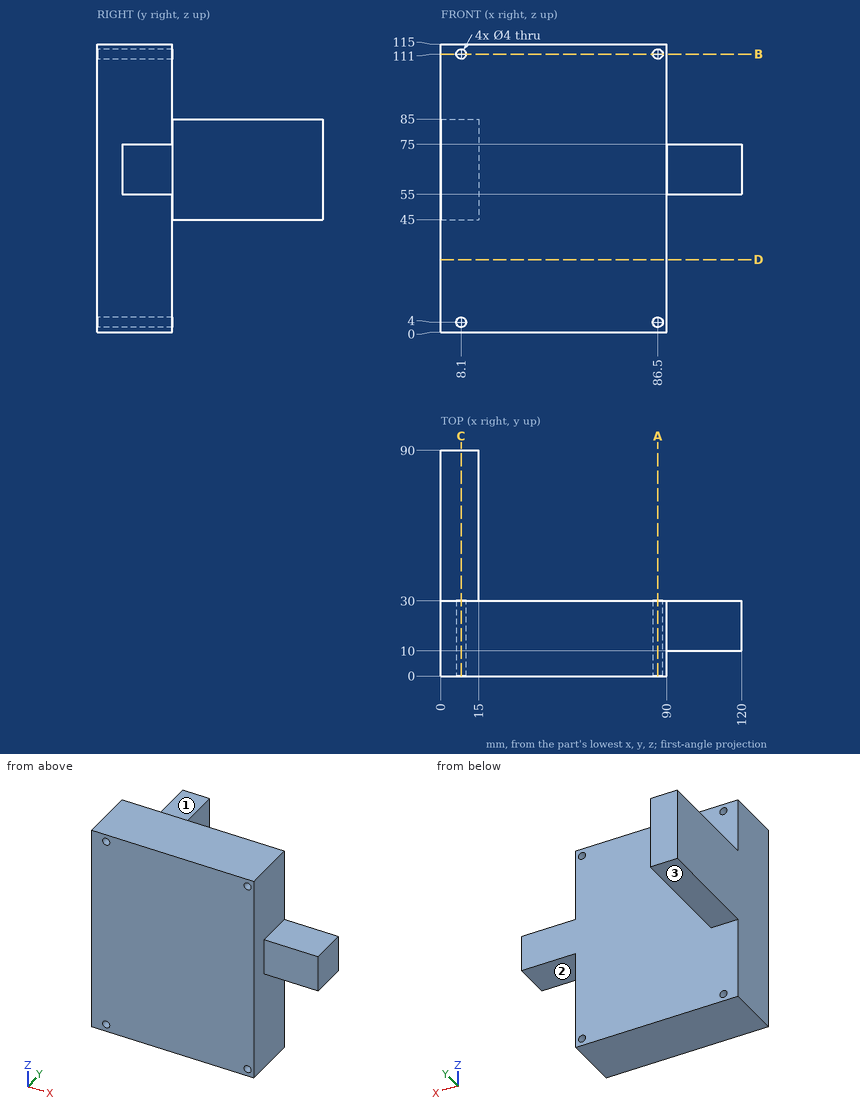
For this review, use the dimensioned drawing (mm, ordinates from the lowest corner) and the shaded views. A direction names the side the tool comes from. Coordinates: 2 decimals unless noted, no trailing zeros. Loops run counter-clockwise (first coordinate to the right, second up) from the corner with the lowest first, then second, coordinate; pieces in that order, holes last. Notation, with made-up numbers: (63.25, -9.75) -> (91.25, -9.75) arc R24 cw to (91.25, 24.25) -> close; hole circle Ø11 at (15.5, 38.5). An arc over 180 degrees is marked (long way). Use a Markdown table: item, result. Add a question column.
1. Add section C-C on x = 8.1. Write out the cut boundary in (y, z), plus the area to 3 significant figures.
2. Add section B-B on z = 111. Write out the cut boundary in (x, y), plus the area to 3 significant figures.
3. To check wall thickness, follow line 1 (Z direction, x = 8, y = 7); line 2 (X direction, y = 18, z = 4); line 3 (Z direction, x = 86, y = 8). State the ranges of each line that lie inside material, in increasing order.
4. Add section D-D on z = 29. Write out the cut boundary in (x, y), plus the area to 3 significant figures.
5. Clearance check with flat-ended pins moving along their axes: pin 1 Ø6 at (y, z) = (40.5, 61) entering from -X; pin 2 Ø22 at (x, z) = (107, 70) entering from -Y; pin 3 Ø4.5 at (x, y) = (5, 46) entering from +Z; pin 4 Ø6 at (x, y) = (112.5, 15) entering from -Z. State where each tip first meets the part, or that it passes through.
6. Add section A-A on x = 86.5. Write out the cut boundary in (y, z).
7. Machinability: for the marked faces 1, 2 and 3, which of the approach directions +Z, -Z, +X, -X, +Y, -Y give a long, thin tool a straight path to every point of the face, cutting with its end or side? Answer none if there is none.
Returned:
| question | item | result |
|---|---|---|
| 1 | outline | (0, 0) -> (30, 0) -> (30, 2) -> (0, 2) -> close; (0, 6) -> (30, 6) -> (30, 45) -> (90, 45) -> (90, 85) -> (30, 85) -> (30, 109) -> (0, 109) -> close; (0, 113) -> (30, 113) -> (30, 115) -> (0, 115) -> close |
| 1 | area | 5,610 mm² |
| 2 | outline | (0, 0) -> (6.1, 0) -> (6.1, 30) -> (0, 30) -> close; (10.1, 0) -> (84.5, 0) -> (84.5, 30) -> (10.1, 30) -> close; (88.5, 0) -> (90, 0) -> (90, 30) -> (88.5, 30) -> close |
| 2 | area | 2,460 mm² |
| 3 | line 1 | z = 0 to 2, 6 to 109, 113 to 115 |
| 3 | line 2 | x = 0 to 6.1, 10.1 to 84.5, 88.5 to 90 |
| 3 | line 3 | z = 0 to 2.06, 5.94 to 109.06, 112.94 to 115 |
| 4 | outline | (0, 0) -> (90, 0) -> (90, 30) -> (0, 30) -> close |
| 4 | area | 2,700 mm² |
| 5 | pin 1 | stops at x = 0 |
| 5 | pin 2 | stops at y = 10 |
| 5 | pin 3 | stops at z = 85 |
| 5 | pin 4 | stops at z = 55 |
| 6 | outline | (0, 0) -> (30, 0) -> (30, 2) -> (0, 2) -> close; (0, 6) -> (30, 6) -> (30, 109) -> (0, 109) -> close; (0, 113) -> (30, 113) -> (30, 115) -> (0, 115) -> close |
| 7 | face 1 | +Z, +X, -X, +Y |
| 7 | face 2 | -Z, +X, +Y, -Y |
| 7 | face 3 | -Z, +X, -X, +Y |
